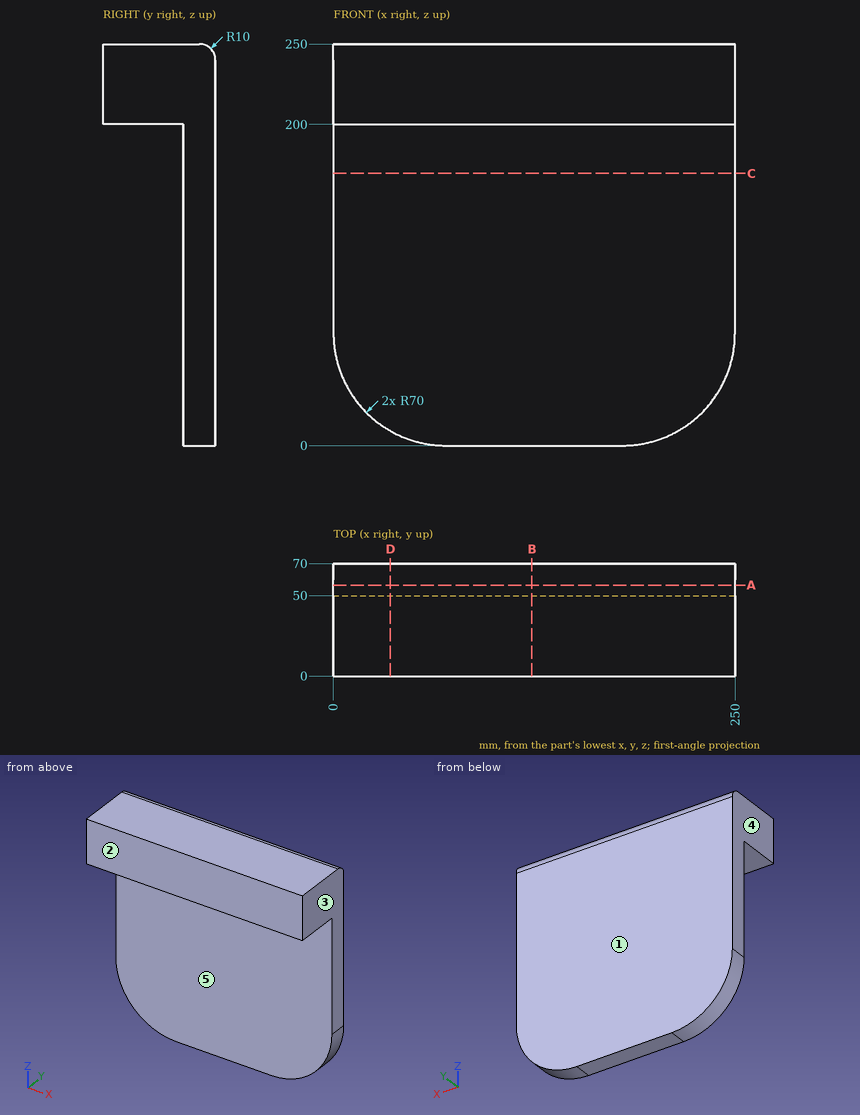
Geometry check sheet. Reference: drawing and pictorial views, mm from the part's lowest x, y, z. A direction names the side the tool comes from. Give positions to 0.01 mm unless a question says otherwise; leave off trailing zeros. Loops run counter-clockwise (first coordinate to the right, second up) from the corner with the lowest first, then second, coordinate; pieces in that order, holes last. Notation, with made-up numbers: (21, -8) - (55, -8) arc R27 ccw to (55, 31) - close; hole circle Ø3 at (12.5, 73). An arc over 180 degrees is marked (long way). Use CSV: the item, a comma, the result in double quotes. Start each with the question number.
Q1. Section check B-B, the plane x = 123.5. Record the cut outline in (y, z), and give its area (3 significant figures).
Q2. Section check C-C, the plane z = 169.5. Record the cut outline in (x, y), and give its area (3 significant figures).
Q3. Access from +Z, -Z, +X, -X, +Y, -Y to the whole of each face (thin tool, end or side, straight path). Record for the marked faces 4 and 5.
Q4. Section check D-D, the plane x = 35.5. Record the cut outline in (y, z).
Q5. Scan lines: probe 1 along Z at (x, y) = (198, 38); probe 2 along Y at (x, z) = (71, 69.5); probe 3 along X at (y, z) = (65, 44.5). Record each from-to range of solid material in increasing order. Write a range as from..to.
Q6. Section check A-A, the plane y = 56.5. Record the cut outline in (x, z).
Q7. Go/stop test with flat-tipped pins: pin 1 Ø25 at (x, y) = (109, 26) entering from -Z; pin 2 Ø1.5 at (x, z) = (199, 195.5) entering from -Y; pin 3 Ø10 at (x, y) = (40, 49) entering from -Z. Record where each tip stops, or that it passes through.
Q8. Release check for a two-part mould opening along Y. For the marked faces 1, 2 and 3 record: +Y half, -Y half, draft (parallel to the pull), parting line (faces both ways), or undercut.
Findings below:
1,outline,"(0, 200) - (50, 200) - (50, 0) - (70, 0) - (70, 240) arc R10 ccw to (60, 250) - (0, 250) - close"
1,area,"7,480 mm^2"
2,outline,"(0, 50) - (250, 50) - (250, 70) - (0, 70) - close"
2,area,"5,000 mm^2"
3,face 4,"+Z, -Z, -X, +Y, -Y"
3,face 5,"-Z, +X, -X, -Y"
4,outline,"(0, 200) - (50, 200) - (50, 9.09) - (70, 9.09) - (70, 240) arc R10 ccw to (60, 250) - (0, 250) - close"
5,probe 1,"z = 200..250"
5,probe 2,"y = 50..70"
5,probe 3,"x = 4.81..245.19"
6,outline,"(0, 70) arc R70 ccw to (70, 0) - (180, 0) arc R70 ccw to (250, 70) - (250, 250) - (0, 250) - close"
7,pin 1,"stops at z = 200"
7,pin 2,"stops at y = 50"
7,pin 3,"stops at z = 4.66"
8,face 1,"+Y half"
8,face 2,"-Y half"
8,face 3,"draft"
